Here's how the part is built. I have some questions about the finished solid (model axes, mm). Face numbers are marked on the shaded views. A direction names the side the tool comes from. Coordinates: 2 decimals unless noted, no trailing zeros. Write each loop counter-clockwise with the first axis right and the second up, starting at its lowest first coordinate (ties: lowest second). Pieces come first, ordered by that corner, then holes.
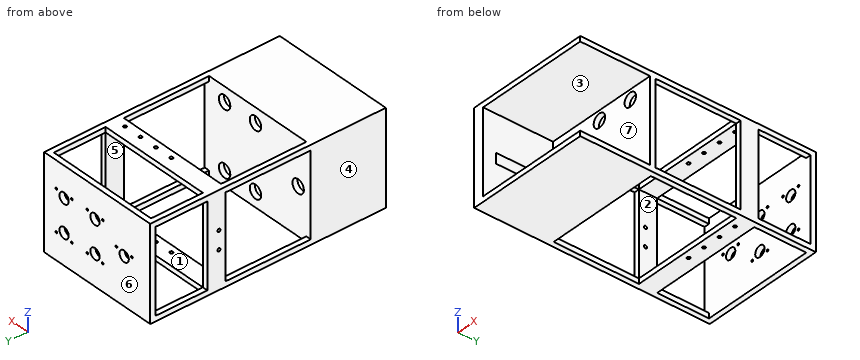
from build123d import *

# Parameters (mm, degrees)
SKETCH1_W           = 240.15
SKETCH1_H           = 180.3
BOSS_EXTRUDE1_DEPTH = 145
SKETCH2_R           = 12.955
CUT_EXTRUDE1_DEPTH  = 120
SKETCH3_W           = 160.42
SKETCH3_H           = 135.06
CUT_EXTRUDE3_DEPTH  = 220
SKETCH9_W           = 240.15
SKETCH9_H           = 180.3
BOSS_EXTRUDE3_DEPTH = 310.134
SKETCH14_R          = 10.5
SKETCH14_R_2        = 2
CUT_EXTRUDE6_DEPTH  = 11
SKETCH15_W          = 220.15
SKETCH15_H          = 100.24
SKETCH15_H_2        = 164.844
CUT_EXTRUDE7_DEPTH  = 181.3
SKETCH16_W          = 160.3
SKETCH16_H          = 100.24
SKETCH16_H_2        = 164.842
CUT_EXTRUDE8_DEPTH  = 241.15
CUT_EXTRUDE9_REACH  = 346.894
SKETCH17_W          = 220.15
SKETCH17_H          = 160.3
SKETCH18_R          = 3
CUT_EXTRUDE10_DEPTH = 249
SKETCH19_R          = 3
CUT_EXTRUDE11_DEPTH = 104


with BuildPart() as part:
    # Sketch1 → Boss-Extrude1 (new body)
    with BuildSketch(Plane(origin=(0, 0, 0), x_dir=(1, 0, 0), z_dir=(0, 1, 0))):
        Rectangle(SKETCH1_W, SKETCH1_H)
    extrude(amount=BOSS_EXTRUDE1_DEPTH)

    # Sketch2 → Cut-Extrude1 (cut)
    with BuildSketch(Plane(origin=(0, 145, 0), x_dir=(1, 0, 0), z_dir=(0, 1, 0))):
        with Locations((75.105, -61.65)):
            Circle(SKETCH2_R)
        with Locations((5.105, -61.65)):
            Circle(SKETCH2_R)
        with Locations((75.105, 61.65)):
            Circle(SKETCH2_R)
        with Locations((5.105, 61.65)):
            Circle(SKETCH2_R)
        with Locations((-91.515, 0)):
            Circle(SKETCH2_R)
    extrude(amount=-CUT_EXTRUDE1_DEPTH, mode=Mode.SUBTRACT)

    # Sketch3 → Cut-Extrude3 (cut)
    with BuildSketch(Plane(origin=(120.075, 0, 0), x_dir=(0, 0, -1), z_dir=(1, 0, 0))):
        with Locations((0, 67.53)):
            Rectangle(SKETCH3_W, SKETCH3_H)
    extrude(amount=-CUT_EXTRUDE3_DEPTH, mode=Mode.SUBTRACT)

    # Sketch9 → Boss-Extrude3 (add)
    with BuildSketch(Plane(origin=(0, 145, 0), x_dir=(1, 0, 0), z_dir=(0, 1, 0))):
        Rectangle(SKETCH9_W, SKETCH9_H)
    extrude(amount=BOSS_EXTRUDE3_DEPTH)

    # Sketch14 → Cut-Extrude6 (cut)
    with BuildSketch(Plane(origin=(0, 455.134, 0), x_dir=(1, 0, 0), z_dir=(0, 1, 0))):
        with Locations((5.105, -31.17)):
            Circle(SKETCH14_R)
        with Locations((75.105, 31.17)):
            Circle(SKETCH14_R)
        with Locations((-61.035, 0)):
            Circle(SKETCH14_R)
        with Locations((75.105, -31.17)):
            Circle(SKETCH14_R)
        with Locations((92.605, -39.14)):
            Circle(SKETCH14_R_2)
        with Locations((57.605, -39.14)):
            Circle(SKETCH14_R_2)
        with Locations((5.105, 31.17)):
            Circle(SKETCH14_R)
        with Locations((92.605, 39.14)):
            Circle(SKETCH14_R_2)
        with Locations((57.605, 39.14)):
            Circle(SKETCH14_R_2)
        with Locations((22.605, -39.14)):
            Circle(SKETCH14_R_2)
        with Locations((-12.395, -39.14)):
            Circle(SKETCH14_R_2)
        with Locations((22.605, 39.14)):
            Circle(SKETCH14_R_2)
        with Locations((-12.395, 39.14)):
            Circle(SKETCH14_R_2)
        with Locations((-43.535, -7.97)):
            Circle(SKETCH14_R_2)
        with Locations((-78.535, -7.97)):
            Circle(SKETCH14_R_2)
    extrude(amount=-CUT_EXTRUDE6_DEPTH, mode=Mode.SUBTRACT)

    # Sketch15 → Cut-Extrude7 (cut, through all)
    with BuildSketch(Plane(origin=(0, 0, -90.15), x_dir=(-1, 0, 0), z_dir=(0, 0, -1))):
        with Locations((0, 395.014)):
            Rectangle(SKETCH15_W, SKETCH15_H)
        with Locations((0, 227.422)):
            Rectangle(SKETCH15_W, SKETCH15_H_2)
    extrude(amount=-CUT_EXTRUDE7_DEPTH, mode=Mode.SUBTRACT)

    # Sketch16 → Cut-Extrude8 (cut, through all)
    with BuildSketch(Plane(origin=(120.075, 0, 0), x_dir=(0, 0, -1), z_dir=(1, 0, 0))):
        with Locations((0, 395.014)):
            Rectangle(SKETCH16_W, SKETCH16_H)
        with Locations((0, 227.421)):
            Rectangle(SKETCH16_W, SKETCH16_H_2)
    extrude(amount=-CUT_EXTRUDE8_DEPTH, mode=Mode.SUBTRACT)

    # Sketch17 → Cut-Extrude9 (cut, up to next)
    with BuildSketch(Plane(origin=(0, 344.894, 0), x_dir=(1, 0, 0), z_dir=(0, 1, 0)), mode=Mode.PRIVATE) as cut_extrude9_sk1:
        Rectangle(SKETCH17_W, SKETCH17_H)
    cut_extrude9_tool1 = extrude(cut_extrude9_sk1.sketch, amount=-CUT_EXTRUDE9_REACH, mode=Mode.PRIVATE) & part.part
    add(cut_extrude9_tool1.solids().sort_by_distance((0, 344.894, 0))[0], mode=Mode.SUBTRACT)

    # Sketch18 → Cut-Extrude10 (cut)
    with BuildSketch(Plane.XY.offset(90.15)):
        with Locations((-12.395, 322.394)):
            Circle(SKETCH18_R)
        with Locations((22.605, 322.394)):
            Circle(SKETCH18_R)
        with Locations((57.605, 322.394)):
            Circle(SKETCH18_R)
        with Locations((92.605, 322.394)):
            Circle(SKETCH18_R)
    extrude(amount=-CUT_EXTRUDE10_DEPTH, mode=Mode.SUBTRACT)

    # Sketch19 → Cut-Extrude11 (cut)
    with BuildSketch(Plane.ZY.offset(120.075)):
        with Locations((-17.5, 322.392)):
            Circle(SKETCH19_R)
        with Locations((17.5, 322.392)):
            Circle(SKETCH19_R)
    extrude(amount=-CUT_EXTRUDE11_DEPTH, mode=Mode.SUBTRACT)


solid = part.part
1. I want a section at B-B (z = 61.65). List the corners of the cut face in (x, y) for me (3 decimals).
2. I want a section at C-C (y = 265). List the corners of the cut face in (x, z) for me (3 decimals).
3. Thinking about a two-plate mould opening in X: for the marked faces 1, 2, 3 and 4, which applies, pulls with the +X half, pulls with the -X half, needs draft (parallel to the pull), parting line crosses it, or undercut?
4. For pin 1 Ø3 at (x, z) = (60.5, 40) entering from -Y; pin 2 Ø23.5 at (x, z) = (75.105, 61.65) entering from -Y, each with a flat end and sliding along its axis, tell me the tip position at first contact or that it passes through.
5. If I drill on line 1 (X direction, y = 453, z = -31) (3 decimals); line 2 (Y direction, x = -77.5, z = 30); line 3 (X direction, y = 143.25, z = -61.65) (3 decimals), over which ranges is the centre line in solid material (lowest first)?
6. I want a section at D-D (x = -85). List the corners of the cut face in (y, z) for me, then the cut area to 3 significant figures.
7. On a 3-axis mill with a long thin cutter (end or side, diameter ignored), from which of +Z, -Z, +X, -X, +Y, -Y can I reach the whole of each face in a straight line? I mean the marked faces 5, 6 and 7. Say none if no direction works.
8. I want a section at A-A (x = 42.5). List the corners of the cut face in (y, z) for me.
Response values:
1. outline: (-120.075, 0) - (-99.925, 0) - (-99.925, 135.06) - (-7.85, 135.06) - (-7.85, 145) - (-120.075, 145) - close; (-120.075, 309.842) - (-110.075, 309.842) - (-110.075, 344.894) - (-120.075, 344.894) - close; (-120.075, 445.134) - (120.075, 445.134) - (120.075, 455.134) - (-120.075, 455.134) - close; (18.06, 135.06) - (62.15, 135.06) - (62.15, 145) - (18.06, 145) - close; (88.06, 135.06) - (120.075, 135.06) - (120.075, 145) - (88.06, 145) - close; (110.075, 309.842) - (120.075, 309.842) - (120.075, 344.894) - (110.075, 344.894) - close
2. outline: (-120.075, -90.15) - (-110.075, -90.15) - (-110.075, -80.15) - (-120.075, -80.15) - close; (-120.075, 80.15) - (-110.075, 80.15) - (-110.075, 90.15) - (-120.075, 90.15) - close; (110.075, -90.15) - (120.075, -90.15) - (120.075, -80.15) - (110.075, -80.15) - close; (110.075, 80.15) - (120.075, 80.15) - (120.075, 90.15) - (110.075, 90.15) - close
3. face 1: undercut
3. face 2: undercut
3. face 3: needs draft
3. face 4: pulls with the -X half
4. pin 1: stops at y = 135.06
4. pin 2: stops at y = 445.13
5. line 1: x = -120.075 to -5.394, 15.604 to 64.606, 85.604 to 120.075
5. line 2: y = 135.06 to 145, 445.13 to 455.13
5. line 3: x = -120.075 to -7.85, 18.06 to 62.15, 88.06 to 120.075
6. outline: (0, -90.15) - (145, -90.15) - (145, -11.2) - (135.06, -11.2) - (135.06, -80.21) - (0, -80.21) - close; (0, 80.21) - (135.06, 80.21) - (135.06, 11.2) - (145, 11.2) - (145, 90.15) - (0, 90.15) - close; (309.84, -90.15) - (344.89, -90.15) - (344.89, -80.15) - (309.84, -80.15) - close; (309.84, 80.15) - (344.89, 80.15) - (344.89, 90.15) - (309.84, 90.15) - close; (445.13, -90.15) - (455.13, -90.15) - (455.13, 90.15) - (445.13, 90.15) - close
6. area: 6,760 mm2
7. face 5: none
7. face 6: +Z, -Z, +X, -X, +Y
7. face 7: +X, -Y
8. outline: (0, -90.15) - (145, -90.15) - (145, 90.15) - (0, 90.15) - (0, 80.21) - (135.06, 80.21) - (135.06, -80.21) - (0, -80.21) - close; (309.84, -90.15) - (344.89, -90.15) - (344.89, -80.15) - (309.84, -80.15) - close; (309.84, 80.15) - (344.89, 80.15) - (344.89, 90.15) - (309.84, 90.15) - close; (445.13, -90.15) - (455.13, -90.15) - (455.13, 90.15) - (445.13, 90.15) - close
